Here's the drawing with two shaded views (mm, measured from the low corner). I have some questions. Round coordinates to 2 decimals unless told otherwise and drop trailing zeros. Order: outer loops, then holes, each group sorted by start corner. A loop starts at its lowest first (then second) coordinate and runs counter-clockwise, first axis right, second up.
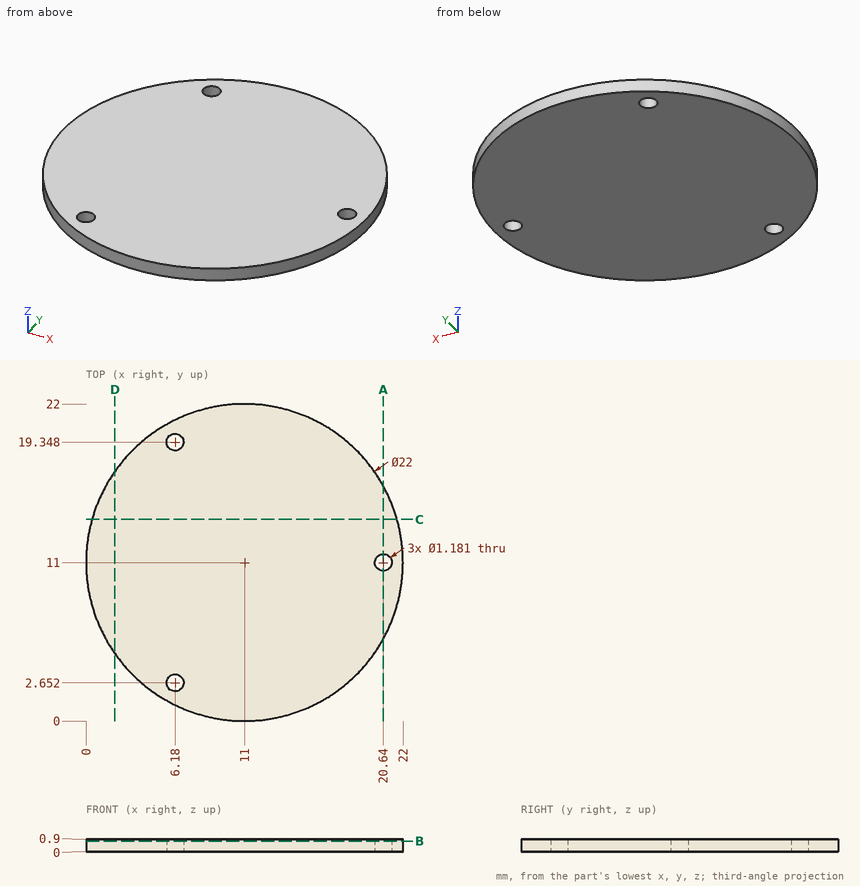
1. If we section it at A-A, the plane x = 20.64: Write out the boundary of the cut face in (y, z).
Evaluation:
outline: (5.7, 0) - (10.41, 0) - (10.41, 0.9) - (5.7, 0.9) - close; (11.59, 0) - (16.3, 0) - (16.3, 0.9) - (11.59, 0.9) - close
2. If we section it at D-D, the plane x = 2: Write out the boundary of the cut face in (y, z) (1 decimal).
Evaluation:
outline: (4.7, 0) - (17.3, 0) - (17.3, 0.9) - (4.7, 0.9) - close
3. I'm going to push a flat-ended pin straight in: P1, Ø1.1, axis at x = 6.18, y = 2.65, coming from the -Z side. Where does the tip first touch, or does it pass through?
Evaluation:
P1: passes through
4. If we section it at C-C, the plane y = 14: Write out the boundary of the cut face in (x, z).
Evaluation:
outline: (0.42, 0) - (21.58, 0) - (21.58, 0.9) - (0.42, 0.9) - close
5. I need wall thicknesses on probe 1 along X at (y, z) = (1.25, 0.85) (1 decimal); probe 2 along X at (y, z) = (17.5, 0.8) (1 decimal); probe 3 along Y at (x, z) = (20.64, 0.5) (1 decimal). Which ranges of each line are inside material? Lowest first, please.
Evaluation:
probe 1: x = 5.9 to 16.1
probe 2: x = 2.1 to 19.9
probe 3: y = 5.7 to 10.4, 11.6 to 16.3
6. If we section it at B-B, the plane z = 0.75: Write out the boundary of the cut face in (x, y).
Evaluation:
outline: circle Ø22 at (11, 11); hole circle Ø1.18 at (6.18, 2.65); hole circle Ø1.18 at (6.18, 19.35); hole circle Ø1.18 at (20.64, 11)
